from build123d import *

# Parameters (mm, degrees)
SKETCH1_R                  = 38.1
BOSS_EXTRUDE1_DEPTH        = 6.35
SKETCH3_R                  = 38.1
SKETCH3_R_2                = 34.925
CUT_EXTRUDE_THIN1_DEPTH    = 3.175
SKETCH8_R                  = 12.7
BOSS_EXTRUDE2_DEPTH        = 25.4
F_1_2_0_5_DIAMETER_HOLE1_D = 12.7
F_10_32_TAPPED_HOLE1_D     = 4.0386
CIRPATTERN1_COUNT          = 6


with BuildPart() as part:
    # Sketch1 → Boss-Extrude1 (new body)
    with BuildSketch(Plane(origin=(0, 0, 0), x_dir=(0, 0, -1), z_dir=(1, 0, 0))):
        Circle(SKETCH1_R)
    extrude(amount=BOSS_EXTRUDE1_DEPTH)

    # Sketch3 → Cut-Extrude-Thin1 (cut)
    with BuildSketch(Plane(origin=(6.35, 0, 0), x_dir=(0, 0, -1), z_dir=(1, 0, 0))):
        Circle(SKETCH3_R)
        Circle(SKETCH3_R_2, mode=Mode.SUBTRACT)
    extrude(amount=-CUT_EXTRUDE_THIN1_DEPTH, mode=Mode.SUBTRACT)

    # Sketch8 → Boss-Extrude2 (add)
    with BuildSketch(Plane.ZY):
        Circle(SKETCH8_R)
    extrude(amount=BOSS_EXTRUDE2_DEPTH)

    # 1/2 (0.5) Diameter Hole1 (through all)
    with Locations(Plane(origin=(6.35, 0, 0), x_dir=(0, 0, -1), z_dir=(1, 0, 0))):
        with Locations((0, 0)):
            Hole(F_1_2_0_5_DIAMETER_HOLE1_D / 2)

    # #10-32 Tapped Hole1 (through all)
    with Locations(Plane.ZY):
        with Locations((0, 23.8125)):
            f_10_32_tapped_hole1 = Hole(F_10_32_TAPPED_HOLE1_D / 2)

    # CirPattern1: #10-32 Tapped Hole1 ×6 about axis
    cirpattern1_axis = Axis((0, 0, 0), (1, 0, 0))
    for i in range(1, CIRPATTERN1_COUNT):
        add(f_10_32_tapped_hole1.rotate(cirpattern1_axis, i * 360 / CIRPATTERN1_COUNT), mode=Mode.SUBTRACT)


solid = part.part
Design review of the part built by this model. Coordinates are the model's own, in mm. A direction names the side the tool comes from. Round coordinates to 2 decimals unless told otherwise and drop trailing zeros. Loops run counter-clockwise (first coordinate to the right, second up) from the corner with the lowest first, then second, coordinate; pieces in that order, holes last. Notation, with made-up numbers: M 19,43.25 L 61,43.25 A14 cw 61,49.25 Z; hole C 81,9.5 d4. An arc over 180 degrees is marked long. Answer as a JSON object with one key per item and string values.
Item 1: We need section A-A on y = 0. Give the boundary of the cut face in (x, z) (3 decimals).
Answer sheet:
{"outline": "M -25.4,-12.7 L 0,-12.7 L 0,-38.1 L 3.175,-38.1 L 3.175,-34.925 L 6.35,-34.925 L 6.35,-6.35 L -25.4,-6.35 Z; M -25.4,6.35 L 6.35,6.35 L 6.35,34.925 L 3.175,34.925 L 3.175,38.1 L 0,38.1 L 0,12.7 L -25.4,12.7 Z"}
Item 2: Wall thickness on L1, parallel to Y at x = 2, z = 0; L2, parallel to Z at x = 3.5, y = 12; L3, parallel to X at y = -20.5, z = -24: over which ranges is each line inside the solid? List them lowest first. Write a range as from..to.
Answer sheet:
{"L1": "y = -38.1..-25.83, -21.79..-6.35, 6.35..21.79, 25.83..38.1", "L2": "z = -32.8..-22.64, -18.61..18.61, 22.64..32.8", "L3": "x = 0..6.35"}
Item 3: We need section B-B on z = 0. Give the boundary of the cut face in (x, y) (3 decimals), and give its area (3 significant figures).
Answer sheet:
{"outline": "M -25.4,-12.7 L 0,-12.7 L 0,-21.793 L 6.35,-21.793 L 6.35,-6.35 L -25.4,-6.35 Z; M -25.4,6.35 L 6.35,6.35 L 6.35,21.793 L 0,21.793 L 0,12.7 L -25.4,12.7 Z; M 0,-38.1 L 3.175,-38.1 L 3.175,-34.925 L 6.35,-34.925 L 6.35,-25.832 L 0,-25.832 Z; M 0,25.832 L 6.35,25.832 L 6.35,34.925 L 3.175,34.925 L 3.175,38.1 L 0,38.1 Z", "area": "654 mm^2"}
Item 4: Clearance check with flat-ended pins moving along their axes: P1, Ø6, axis at x = 0.5, z = -10.5, coming from the +Y side; P2, Ø6.5, axis at y = -11.91, z = -20.62, coming from the -X side; P3, Ø4.5, axis at y = 11.91, z = 20.62, coming from the +X side; P4, Ø12, axis at x = -16, z = -5.5, coming from the +Y side. State where each tip first meets the part, or that it passes through.
Answer sheet:
{"P1": "stops at y = 37.35", "P2": "stops at x = 0", "P3": "stops at x = 6.35", "P4": "stops at y = 12.7"}
Item 5: We need section D-D on x = -6. Give the boundary of the cut face in (y, z), and give its area (3 significant figures).
Answer sheet:
{"outline": "C 0,0 d25.4; hole C 0,0 d12.7", "area": "380 mm^2"}
Item 6: The part is to be moulded in two halves that separate along Z. For faces 4 (the cylindrical face through (-9.75, -6.2, -1.38)), 5 (the cylindrical face through (4.785, -21.251, 27.715)), 6 (the flat face through (0, 1, -16)), say which applies: pulls with the +Z half, pulls with the -Z half, needs draft (parallel to the pull), parting line crosses it, or undercut.
Answer sheet:
{"face 4": "undercut", "face 5": "parting line crosses it", "face 6": "needs draft"}
Item 7: We need section C-C on y = -30.5. Give the boundary of the cut face in (x, z) (3 decimals), and give its area (3 significant figures).
Answer sheet:
{"outline": "M 0,-22.833 L 3.175,-22.833 L 3.175,-17.015 L 6.35,-17.015 L 6.35,17.015 L 3.175,17.015 L 3.175,22.833 L 0,22.833 Z", "area": "253 mm^2"}
Item 8: Machinability: for faces 1 (the flat face through (3.175, -31, -17)), 2 (the cylindrical face through (-12.52, -12.4, -2.75)), 3 (the cylindrical face through (3.219, -13.878, -20.184)), which of the approach directions +Z, -Z, +X, -X, +Y, -Y give a long, thin tool a straight path to every point of the face, cutting with its end or side? Answer none if there is none.
Answer sheet:
{"face 1": "+X", "face 2": "-X", "face 3": "+X, -X"}
